Design review of the part shown in the three views and the two pictorial views. Dimensions are in mm from the part's minimum x, y and z. Give positions to 0.01 mm unless a question says otherwise; leave off trailing zeros. Order: outer loops, then holes, each group sorted by start corner. A loop starts at its lowest first (then second) coordinate and runs counter-clockwise, first axis right, second up.
Item 1: For probe 1 along Y at (x, z) = (76.2, 10); probe 2 along Y at (x, z) = (73, 8.5); probe 3 along X at (y, z) = (20, 3.5), list the stretches that pass through material, from the lowest coordinate up.
Item 2: Consider section A-A (x = 76.2). Give the boundary of the cut face in (y, z), plus the area to 3 significant figures.
Item 3: The part is to be moulded in two halves that separate along Y. For the marked faces 1, 2, 3 and 4, say which applies: released by +Y, released by -Y, zero draft, split by the parting line, or undercut.
Item 4: Consider section C-C (z = 7.75). Give the boundary of the cut face in (x, y).
Item 5: Consider section B-B (y = 25.4). Give the boundary of the cut face in (x, z), plus the area to 3 significant figures.
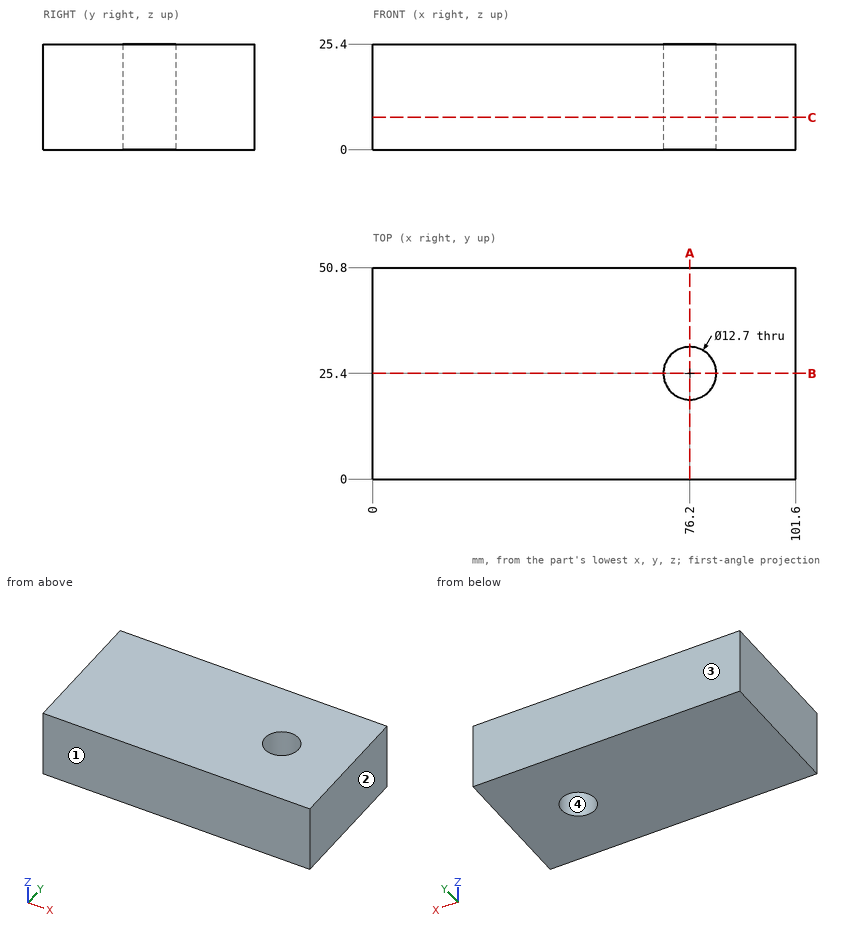
Resolved:
1. probe 1: y = 0 to 19.05, 31.75 to 50.8
1. probe 2: y = 0 to 19.92, 30.88 to 50.8
1. probe 3: x = 0 to 72.86, 79.54 to 101.6
2. outline: (0, 0) - (19.05, 0) - (19.05, 25.4) - (0, 25.4) - close; (31.75, 0) - (50.8, 0) - (50.8, 25.4) - (31.75, 25.4) - close
2. area: 968 mm2
3. face 1: released by -Y
3. face 2: zero draft
3. face 3: released by +Y
3. face 4: undercut
4. outline: (0, 0) - (101.6, 0) - (101.6, 50.8) - (0, 50.8) - close; hole circle Ø12.7 at (76.2, 25.4)
5. outline: (0, 0) - (69.85, 0) - (69.85, 25.4) - (0, 25.4) - close; (82.55, 0) - (101.6, 0) - (101.6, 25.4) - (82.55, 25.4) - close
5. area: 2,260 mm2
